from build123d import *

# Parameters (mm, degrees)
SKETCH1_W           = 16
SKETCH1_H           = 10
BOSS_EXTRUDE1_DEPTH = 3
CUT_EXTRUDE1_REACH  = 11.899
SKETCH2_R           = 1.5
FILLET1_R           = 5


with BuildPart() as part:
    # Sketch1 → Boss-Extrude1 (new body)
    with BuildSketch(Plane(origin=(0, 0, 0), x_dir=(1, 0, 0), z_dir=(0, 1, 0))):
        Rectangle(SKETCH1_W, SKETCH1_H)
    extrude(amount=BOSS_EXTRUDE1_DEPTH)

    # Sketch2 → Cut-Extrude1 (cut, up to next)
    with BuildSketch(Plane(origin=(0, 0, 0), x_dir=(1, 0, 0), z_dir=(0, 1, 0)), mode=Mode.PRIVATE) as cut_extrude1_sk1:
        with Locations(Location((0, -1, 0), (0, 0, 90))):
            Circle(SKETCH2_R)
    cut_extrude1_tool1 = extrude(cut_extrude1_sk1.sketch, amount=CUT_EXTRUDE1_REACH, mode=Mode.PRIVATE) & part.part
    add(cut_extrude1_tool1.solids().sort_by_distance((0, 0, 1))[0], mode=Mode.SUBTRACT)

    # Fillet1
    fillet1_edges = [part.edges().sort_by_distance(p)[0] for p in [
        (8, 1.5, 5),
        (-8, 1.5, 5),
    ]]
    fillet(fillet1_edges, radius=FILLET1_R)


solid = part.part
Could you check a few things on this model? Use its own coordinates, in mm. Give positions to 0.01 mm unless a question says otherwise; leave off trailing zeros. Loops run counter-clockwise (first coordinate to the right, second up) from the corner with the lowest first, then second, coordinate; pieces in that order, holes last. Notation, with made-up numbers: (-19.5, -18) -> (9.5, -18) arc R17 cw to (9.5, 2) -> close; hole circle Ø8 at (-5.5, 76). An arc over 180 degrees is marked (long way). Return JSON: item names as keys, results as strings.
Item 1: I'm going to push a flat-ended pin straight in: pin 1 (1.5 mm diameter, centred on y = 1, z = 3, fed in from +X). Where does the tip first touch, or does it pass through?
Geometry results:
{"pin 1": "stops at x = 7.47"}
Item 2: If we section it at A-A on x = 0: List the corners of the cut face in (y, z) for me, plus the area to 3 significant figures.
Geometry results:
{"outline": "(0, -5) -> (3, -5) -> (3, -0.5) -> (0, -0.5) -> close; (0, 2.5) -> (3, 2.5) -> (3, 5) -> (0, 5) -> close", "area": "21.0 mm²"}
Item 3: If we section it at D-D on z = 4: List the corners of the cut face in (x, y) for me, plus the area to 3 significant figures.
Geometry results:
{"outline": "(-6, 0) -> (6, 0) -> (6, 3) -> (-6, 3) -> close", "area": "36.0 mm²"}
Item 4: We'd pull the mould along X, two halves only. Please class faces 1 (the flat face through (0, 1, 5)), 2 (the cylindrical face through (-7, 2, 3)), 3 (the cylindrical face through (-1.01, 1.48, 2.11)): +X half, -X half, draft (parallel to the pull), parting line (faces both ways), or undercut.
Geometry results:
{"face 1": "draft", "face 2": "-X half", "face 3": "undercut"}
Item 5: If we section it at C-C on z = 1.5: List the corners of the cut face in (x, y) for me.
Geometry results:
{"outline": "(-7.77, 0) -> (-1.41, 0) -> (-1.41, 3) -> (-7.77, 3) -> close; (1.41, 0) -> (7.77, 0) -> (7.77, 3) -> (1.41, 3) -> close"}
Item 6: If we section it at B-B on y = 1.2: List the corners of the cut face in (x, z) for me.
Geometry results:
{"outline": "(-8, -5) -> (8, -5) -> (8, 0) arc R5 ccw to (3, 5) -> (-3, 5) arc R5 ccw to (-8, 0) -> close; hole circle Ø3 at (0, 1)"}
Item 7: I need wall thicknesses on L1, parallel to X at y = 0.85, z = 1; L2, parallel to X at y = 0.4, z = 2.25; L3, parallel to Z at x = -0.5, y = 1.45. Which ranges of each line are inside material? Lowest first, please. Write a range as from..to.
Geometry results:
{"L1": "x = -7.9..-1.5, 1.5..7.9", "L2": "x = -7.47..-0.83, 0.83..7.47", "L3": "z = -5..-0.41, 2.41..5"}
